Geometry check sheet. Reference: the model listing, model coordinates, mm. A direction names the side the tool comes from. Coordinates: 2 decimals unless noted, no trailing zeros. Loops run counter-clockwise (first coordinate to the right, second up) from the corner with the lowest first, then second, coordinate; pieces in that order, holes last. Notation, with made-up numbers: M -15.5,-10.75 L -3.5,-10.75 A10 cw -3.5,4.25 Z; hole C -32,67 d7. An arc over 180 degrees is marked long. One line per question, with ' | ' between items. Start each with the question number.
from build123d import *

# Parameters (mm, degrees)
F0_R          = 8.5
F1_DEPTH      = 21
F2_R          = 6.125
F3_DEPTH      = 8.501
F3_DEPTH_BACK = 25.4
F4_R          = 1.5
F5_W          = 5.8
F5_H          = 2.9
F6_DEPTH      = 25.4
F6_DEPTH_BACK = 25.4
F7_R          = 1.778
F8_DEPTH      = 10


with BuildPart() as f1:
    # F0 (on Top) → F1 (new body)
    with BuildSketch(Plane.XY):
        Circle(F0_R)
    extrude(amount=F1_DEPTH)

    # F2 (on Right) → F3 (cut, two sides)
    with BuildSketch(Plane.YZ) as f3_sk:
        with Locations((0, 8.625)):
            Circle(F2_R)
    extrude(amount=-F3_DEPTH, mode=Mode.SUBTRACT)
    extrude(f3_sk.sketch, amount=F3_DEPTH_BACK, mode=Mode.SUBTRACT)

    # F4
    f4_edges = [f1.edges().sort_by_distance(p)[0] for p in [
        (-8.5, 0, 0),
        (-8.5, 0, 21),
    ]]
    fillet(f4_edges, radius=F4_R)

    # F5 (on Right) → F6 (cut, two sides)
    with BuildSketch(Plane.YZ) as f6_sk:
        with Locations((0, 17.05)):
            Rectangle(F5_W, F5_H)
    extrude(amount=-F6_DEPTH, mode=Mode.SUBTRACT)
    extrude(f6_sk.sketch, amount=F6_DEPTH_BACK, mode=Mode.SUBTRACT)

    # F7 (on face) → F8 (cut)
    with BuildSketch(Plane.XY.offset(21)):
        Circle(F7_R)
    extrude(amount=-F8_DEPTH, mode=Mode.SUBTRACT)


solid = f1.part
1. Draft check along Y on faces 3 (the flat face through (1.5, -1.5, 21)), 4 (the cylindrical face through (-1.41, -1.08, 15.05)), 5 (the cylindrical face through (3.92, -7.54, 10.37)). Enter one of: +Y half, -Y half, draft (parallel to the pull), parting line (faces both ways), or undercut.
2. Depth check by flat-ended pin: pin 1 Ø3 at (x, z) = (6, 16.5) entering from +Y; pin 2 Ø0.9 at (x, z) = (-4.5, 17.5) entering from +Y; pin 3 Ø2.5 at (x, z) = (-3.5, 16.5) entering from -Y. Enter the tip coordinate at first touch or a pass-through.
3. Tool access check on faces 1 (the cylindrical face through (-0.385, -1.736, 19.768)), 2 (the flat face through (0, 0, 0)). Record the directions out of +Z, -Z, +X, -X, +Y, -Y that give a thin tool (end or side, any length) a straight path to the whole face; none if there is none.
4. Sectioned sample at D-D (z = 5.5). Record the cut outline in (x, y).
5. Sectioned sample at C-C (x = 5.25). State how many separate pieces and enclosed holes the cut face has, and give its area (3 significant figures).
6. Thickness scan on line 1 (Z direction, x = 4.25, y = 0); line 2 (X direction, y = 0, z = 15.25); line 3 (Y direction, x = 5.75, z = 3.25). Record the ranges inside material, lowest first.
7. Sectioned sample at A-A (y = 0). Record the cut outline in (x, z), and give its area (3 significant figures).
8. Sectioned sample at B-B (z = 10). Record the cut outline in (x, y), and give its area (3 significant figures).
Result:
1) face 3: draft | face 4: undercut | face 5: parting line
2) pin 1: stops at y = 7.21 | pin 2: stops at y = 7.47 | pin 3: stops at y = -8.2
3) face 1: +Z | face 2: -Z, +X, -X, +Y, -Y
4) outline: M -6.67,-5.27 A8.5 ccw 6.67,-5.27 Z; M -6.67,5.27 L 6.67,5.27 A8.5 ccw Z
5) separate pieces: 1 | enclosed holes: 2 | area: 144 mm2
6) line 1: z = 0 to 2.5, 14.75 to 15.6, 18.5 to 21 | line 2: x = -8.5 to -1.78, 1.78 to 8.5 | line 3: y = -6.26 to -2.94, 2.94 to 6.26
7) outline: M -8.5,1.5 A1.5 ccw -7,0 L 7,0 A1.5 ccw 8.5,1.5 L 8.5,2.5 L -8.5,2.5 Z; M -8.5,14.75 L -1.78,14.75 L -1.78,15.6 L -8.5,15.6 Z; M -8.5,18.5 L -1.78,18.5 L -1.78,21 L -7,21 A1.5 ccw -8.5,19.5 Z; M 1.78,14.75 L 8.5,14.75 L 8.5,15.6 L 1.78,15.6 Z; M 1.78,18.5 L 8.5,18.5 L 8.5,19.5 A1.5 ccw 7,21 L 1.78,21 Z | area: 85.6 mm2
8) outline: M -6.05,-5.97 A8.5 ccw 6.05,-5.97 Z; M -6.05,5.97 L 6.05,5.97 A8.5 ccw Z | area: 42.2 mm2
